Read the model definition and answer for the solid it produces. Units are mm, in the model's axes. A direction names the side the tool comes from. Coordinates: 2 decimals unless noted, no trailing zeros. Write each loop counter-clockwise with the first axis right and the second up, starting at its lowest first coordinate (ties: lowest second). Pieces come first, ordered by that corner, then holes.
Item 1: Section D-D (z = -10) is taken. Give the vertices of the cut face in (x, y), then the cut area to 3 significant figures.
Item 2: Section B-B (z = -81) is taken. Give the vertices of the cut face in (x, y).
Item 3: Each of these flat-tipped pins is pushed along its axis until it touches: P1, Ø13, axis at x = 9.5, z = -11, coming from the -Y side; P2, Ø1.8, axis at x = 164.5, y = 8, coming from the +Z side; P3, Ø4, axis at x = 76, y = 4.5, coming from the +Z side. Where does it stop, or does it pass through?
Item 4: Section C-C (y = 4) is taken. Give the vertices of the cut face in (x, z), then the cut area to 3 significant figures.
Item 5: Determine the mould class of faces 6 (the face through (10, 16, -16)), 7 (the face through (155, 10, -44)), 8 (the face through (8.331, 8.526, -2.028)) for opening direction Y: released by +Y, released by -Y, zero draft, split by the parting line, or undercut.
Item 6: Section A-A (x = 100) is taken. Give the vertices of the cut face in (y, z).
Item 7: Straight lines are drawn through the part: probe 1 along X at (y, z) = (3.75, -32.5); probe 2 along Y at (x, z) = (10, -1); probe 3 along Y at (x, z) = (75, -97.3). For each, find the intervals that lie inside material, in ascending order.
Item 8: A tool of negligible diameter and unlimited length cuts with its end or side. For faces 1 (the face through (73.331, 10.526, -98.028)), 2 (the face through (159, 8, -16)), 3 (the face through (20, 10, -42)), 4 (the face through (89, 10, -100)), 5 (the face through (166.669, 8.526, -2.028)), from which of +Z, -Z, +X, -X, +Y, -Y can it reach the whole face along a straight path? Write none if from no direction.
from build123d import *

# Parameters (mm, degrees)
BOSS_EXTRUDE1_DEPTH = 20
FILLET1_R           = 10
SKETCH2_R           = 1.75
CUT_EXTRUDE1_DEPTH  = 203.546291005
SKETCH3_W           = 12
SKETCH3_H           = 24
CUT_EXTRUDE2_DEPTH  = 16
SKETCH4_R           = 1.75
CUT_EXTRUDE3_DEPTH  = 201.601595208
SKETCH6_W           = 12
SKETCH6_H           = 16
BOSS_EXTRUDE2_DEPTH = 0.56


with BuildPart() as part:
    # Sketch1 → Boss-Extrude1 (new body)
    with BuildSketch(Plane(origin=(0, 0, 0), x_dir=(1, 0, 0), z_dir=(0, 1, 0))):
        Polygon((0, 0), (20, 0), (20, 96), (155, 96), (155, 0), (175, 0), (175, 100), (0, 100), align=None)
    extrude(amount=BOSS_EXTRUDE1_DEPTH)

    # Fillet1
    fillet1_edges = [part.edges().sort_by_distance(p)[0] for p in [
        (0, 10, -100),
        (175, 10, -100),
        (155, 10, -96),
        (20, 10, -96),
    ]]
    fillet(fillet1_edges, radius=FILLET1_R)

    # Sketch2 → Cut-Extrude1 (cut, through all)
    with BuildSketch(Plane(origin=(0, 0, -100), x_dir=(-1, 0, 0), z_dir=(0, 0, -1))):
        with Locations((-100, 10)):
            Circle(SKETCH2_R)
        with Locations((-75, 10)):
            Circle(SKETCH2_R)
    extrude(amount=-CUT_EXTRUDE1_DEPTH, mode=Mode.SUBTRACT)

    # Sketch3 → Cut-Extrude2 (cut)
    with BuildSketch(Plane.XZ):
        with Locations((10, -16)):
            Rectangle(SKETCH3_W, SKETCH3_H)
    cut_extrude2 = extrude(amount=-CUT_EXTRUDE2_DEPTH, mode=Mode.SUBTRACT)

    # Sketch4 → Cut-Extrude3 (cut, through all)
    with BuildSketch(Plane(origin=(0, 0, -4), x_dir=(-1, 0, 0), z_dir=(0, 0, -1))):
        with Locations((-10, 8)):
            Circle(SKETCH4_R)
    cut_extrude3 = extrude(amount=-CUT_EXTRUDE3_DEPTH, mode=Mode.SUBTRACT)

    # Mirror1: Cut-Extrude2, Cut-Extrude3 across plane
    add(cut_extrude2.mirror(Plane(origin=(87.5, 0, 0), x_dir=(0, 0, 1), z_dir=(1, 0, 0))), mode=Mode.SUBTRACT)
    add(cut_extrude3.mirror(Plane(origin=(87.5, 0, 0), x_dir=(0, 0, 1), z_dir=(1, 0, 0))), mode=Mode.SUBTRACT)

    # Sketch6 → Boss-Extrude2 (add)
    with BuildSketch(Plane(origin=(0, 0, -4), x_dir=(-1, 0, 0), z_dir=(0, 0, -1))):
        with Locations((-10, 8)):
            Rectangle(SKETCH6_W, SKETCH6_H)
    boss_extrude2 = extrude(amount=BOSS_EXTRUDE2_DEPTH)

    # Mirror2: Boss-Extrude2 across plane
    add(boss_extrude2.mirror(Plane(origin=(87.5, 0, 0), x_dir=(0, 0, 1), z_dir=(1, 0, 0))))


solid = part.part
Established:
1. outline: (0, 0) - (4, 0) - (4, 16) - (16, 16) - (16, 0) - (20, 0) - (20, 20) - (0, 20) - close; (155, 0) - (159, 0) - (159, 16) - (171, 16) - (171, 0) - (175, 0) - (175, 20) - (155, 20) - close
1. area: 416 mm2
2. outline: (0, 0) - (20, 0) - (20, 20) - (0, 20) - close; (155, 0) - (175, 0) - (175, 20) - (155, 20) - close
3. P1: stops at y = 0
3. P2: stops at z = -4
3. P3: stops at z = -96
4. outline: (0, -90) arc R10 ccw to (10, -100) - (165, -100) arc R10 ccw to (175, -90) - (175, 0) - (155, 0) - (155, -86) arc R10 cw to (145, -96) - (30, -96) arc R10 cw to (20, -86) - (20, 0) - (0, 0) - close; hole (4, -28) - (16, -28) - (16, -4.56) - (4, -4.56) - close; hole (159, -28) - (171, -28) - (171, -4.56) - (159, -4.56) - close
4. area: 3,980 mm2
5. face 6: released by -Y
5. face 7: zero draft
5. face 8: undercut
6. outline: (0, -100) - (8.25, -100) - (8.25, -96) - (0, -96) - close; (11.75, -100) - (20, -100) - (20, -96) - (11.75, -96) - close
7. probe 1: x = 0 to 20, 155 to 175
7. probe 2: y = 0 to 6.25, 9.75 to 20
7. probe 3: y = 0 to 8.25, 11.75 to 20
8. face 1: +Z, -Z
8. face 2: -Y
8. face 3: +Z, +Y, -Y
8. face 4: -Z, +X, -X, +Y, -Y
8. face 5: +Z
